from build123d import *

# Parameters (mm, degrees)
SKETCH1_R           = 2.1463
BOSS_EXTRUDE1_DEPTH = 102.5


with BuildPart() as part:
    # Sketch1 → Boss-Extrude1 (new, symmetric)
    with BuildSketch(Plane.XY):
        with BuildLine():
            Line((-9.9949, 7.9883), (-9.9949, 3.2893))
            ThreePointArc((-9.9949, 3.2893), (-9.76427588, 2.73252412), (-9.2075, 2.5019))
            Line((-9.2075, 2.5019), (-8.4963, 2.5019))
            ThreePointArc((-8.4963, 2.5019), (-8.280773853, 2.591173853), (-8.1915, 2.8067))
            Line((-8.1915, 2.8067), (-8.1915, 4.9149))
            ThreePointArc((-8.1915, 4.9149), (-7.674065253, 5.689295824), (-6.760603096, 5.507596904))
            Line((-6.760603096, 5.507596904), (-4.505765747, 3.252759555))
            ThreePointArc((-4.505765747, 3.252759555), (-3.856054457, 2.280397894), (-3.627906192, 1.133419111))
            Line((-3.627906192, 1.133419111), (-3.627906192, -1.133419111))
            ThreePointArc((-3.627906192, -1.133419111), (-3.856054457, -2.280397894), (-4.505765747, -3.252759555))
            Line((-4.505765747, -3.252759555), (-6.760603096, -5.507596904))
            ThreePointArc((-6.760603096, -5.507596904), (-7.674065253, -5.689295824), (-8.1915, -4.9149))
            Line((-8.1915, -4.9149), (-8.1915, -2.8067))
            ThreePointArc((-8.1915, -2.8067), (-8.280773853, -2.591173853), (-8.4963, -2.5019))
            Line((-8.4963, -2.5019), (-9.2075, -2.5019))
            ThreePointArc((-9.2075, -2.5019), (-9.76427588, -2.73252412), (-9.9949, -3.2893))
            Line((-9.9949, -3.2893), (-9.9949, -7.9883))
            ThreePointArc((-9.9949, -7.9883), (-9.407180467, -9.407180467), (-7.9883, -9.9949))
            Line((-7.9883, -9.9949), (-3.2893, -9.9949))
            ThreePointArc((-3.2893, -9.9949), (-2.73252412, -9.76427588), (-2.5019, -9.2075))
            Line((-2.5019, -9.2075), (-2.5019, -8.4963))
            ThreePointArc((-2.5019, -8.4963), (-2.591173853, -8.280773853), (-2.8067, -8.1915))
            Line((-2.8067, -8.1915), (-4.9149, -8.1915))
            ThreePointArc((-4.9149, -8.1915), (-5.689295824, -7.674065253), (-5.507596904, -6.760603096))
            Line((-5.507596904, -6.760603096), (-3.252759555, -4.505765747))
            ThreePointArc((-3.252759555, -4.505765747), (-2.280397894, -3.856054457), (-1.133419111, -3.627906192))
            Line((-1.133419111, -3.627906192), (1.133419111, -3.627906192))
            ThreePointArc((1.133419111, -3.627906192), (2.280397894, -3.856054457), (3.252759555, -4.505765747))
            Line((3.252759555, -4.505765747), (5.507596904, -6.760603096))
            ThreePointArc((5.507596904, -6.760603096), (5.689295824, -7.674065253), (4.9149, -8.1915))
            Line((4.9149, -8.1915), (2.8067, -8.1915))
            ThreePointArc((2.8067, -8.1915), (2.591173853, -8.280773853), (2.5019, -8.4963))
            Line((2.5019, -8.4963), (2.5019, -9.2075))
            ThreePointArc((2.5019, -9.2075), (2.73252412, -9.76427588), (3.2893, -9.9949))
            Line((3.2893, -9.9949), (7.9883, -9.9949))
            ThreePointArc((7.9883, -9.9949), (9.407180467, -9.407180467), (9.9949, -7.9883))
            Line((9.9949, -7.9883), (9.9949, -3.2893))
            ThreePointArc((9.9949, -3.2893), (9.76427588, -2.73252412), (9.2075, -2.5019))
            Line((9.2075, -2.5019), (8.4963, -2.5019))
            ThreePointArc((8.4963, -2.5019), (8.280773853, -2.591173853), (8.1915, -2.8067))
            Line((8.1915, -2.8067), (8.1915, -4.9149))
            ThreePointArc((8.1915, -4.9149), (7.674065253, -5.689295824), (6.760603096, -5.507596904))
            Line((6.760603096, -5.507596904), (4.505765747, -3.252759555))
            ThreePointArc((4.505765747, -3.252759555), (3.856054457, -2.280397894), (3.627906192, -1.133419111))
            Line((3.627906192, -1.133419111), (3.627906192, 1.133419111))
            ThreePointArc((3.627906192, 1.133419111), (3.856054457, 2.280397894), (4.505765747, 3.252759555))
            Line((4.505765747, 3.252759555), (6.760603096, 5.507596904))
            ThreePointArc((6.760603096, 5.507596904), (7.674065253, 5.689295824), (8.1915, 4.9149))
            Line((8.1915, 4.9149), (8.1915, 2.8067))
            ThreePointArc((8.1915, 2.8067), (8.280773853, 2.591173853), (8.4963, 2.5019))
            Line((8.4963, 2.5019), (9.2075, 2.5019))
            ThreePointArc((9.2075, 2.5019), (9.76427588, 2.73252412), (9.9949, 3.2893))
            Line((9.9949, 3.2893), (9.9949, 7.9883))
            ThreePointArc((9.9949, 7.9883), (9.407180467, 9.407180467), (7.9883, 9.9949))
            Line((7.9883, 9.9949), (3.2893, 9.9949))
            ThreePointArc((3.2893, 9.9949), (2.73252412, 9.76427588), (2.5019, 9.2075))
            Line((2.5019, 9.2075), (2.5019, 8.4963))
            ThreePointArc((2.5019, 8.4963), (2.591173853, 8.280773853), (2.8067, 8.1915))
            Line((2.8067, 8.1915), (4.9149, 8.1915))
            ThreePointArc((4.9149, 8.1915), (5.689295824, 7.674065253), (5.507596904, 6.760603096))
            Line((5.507596904, 6.760603096), (3.252759555, 4.505765747))
            ThreePointArc((3.252759555, 4.505765747), (2.280397894, 3.856054457), (1.133419111, 3.627906192))
            Line((1.133419111, 3.627906192), (-1.133419111, 3.627906192))
            ThreePointArc((-1.133419111, 3.627906192), (-2.280397894, 3.856054457), (-3.252759555, 4.505765747))
            Line((-3.252759555, 4.505765747), (-5.507596904, 6.760603096))
            ThreePointArc((-5.507596904, 6.760603096), (-5.689295824, 7.674065253), (-4.9149, 8.1915))
            Line((-4.9149, 8.1915), (-2.8067, 8.1915))
            ThreePointArc((-2.8067, 8.1915), (-2.591173853, 8.280773853), (-2.5019, 8.4963))
            Line((-2.5019, 8.4963), (-2.5019, 9.2075))
            ThreePointArc((-2.5019, 9.2075), (-2.73252412, 9.76427588), (-3.2893, 9.9949))
            Line((-3.2893, 9.9949), (-7.9883, 9.9949))
            ThreePointArc((-7.9883, 9.9949), (-9.407180467, 9.407180467), (-9.9949, 7.9883))
        make_face()
        with Locations(Location((0, 0, 0), (0, 0, 180))):
            Circle(SKETCH1_R, mode=Mode.SUBTRACT)
    extrude(amount=BOSS_EXTRUDE1_DEPTH, both=True)


solid = part.part
Source: CAD feature listing. Evaluate the final solid. Frame: model axes, mm. Coordinates: 2 decimals unless noted, no trailing zeros. Answer in a Markdown table with one row per item. Add a question column.
Q1. Ray query, line 1 along X through (y, z) = (5, -1); line 2 along Y through (x, z) = (0, -46); line 3 along X through (y, z) = (-6.75, -43). Return the intervals inside material, ascending.
Q2. Pull-direction query (X, two-part tool) for faces 1 (the face through (-9.995, -6, 1)), 2 (the face through (-0.1, 2.4, 102.5)), 3 (the face through (1.7, 1.31, -1.44)), 4 (the face through (9.995, -6, 1)); classes: pulls with the +X half, pulls with the -X half, needs draft (parallel to the pull), parting line crosses it, or undercut.
Q3. Contact query for flat-ended pins moving along their axis: pin 1 Ø0.7 at (y, z) = (0, 39.5) entering from +X; pin 2 Ø0.8 at (y, z) = (9, 22.5) entering from +X; pin 3 Ø1.1 at (x, z) = (-0.5, 28) entering from +Y; pin 4 Ø1 at (x, y) = (5, -1.5) entering from +Z. Output: stop coordinate, or through.
Computed values:
| question | item | result |
|---|---|---|
| 1 | line 1 | x = -9.99 to -8.19, -6.25 to -3.75, 3.75 to 6.25, 8.19 to 9.99 |
| 1 | line 2 | y = -3.63 to -2.15, 2.15 to 3.63 |
| 1 | line 3 | x = -9.99 to -5.5, 5.5 to 9.99 |
| 2 | face 1 | pulls with the -X half |
| 2 | face 2 | needs draft |
| 2 | face 3 | undercut |
| 2 | face 4 | pulls with the +X half |
| 3 | pin 1 | stops at x = 3.63 |
| 3 | pin 2 | stops at x = 9.9 |
| 3 | pin 3 | stops at y = 3.63 |
| 3 | pin 4 | passes through |
